from build123d import *

# Parameters (mm, degrees)
F0_W     = 5
F0_H     = 30
F1_DEPTH = 6
F2_R     = 0.948442
F3_DEPTH = 1
F4_R     = 1.863501
F5_DEPTH = 5.001


with BuildPart() as f1:
    # F0 (on Front) → F1 (new body)
    with BuildSketch(Plane.XZ):
        with Locations((2.5, 0)):
            Rectangle(F0_W, F0_H)
    extrude(amount=F1_DEPTH)

    # F2 (on face) → F3 (cut)
    with BuildSketch(Plane.YZ.offset(5)):
        with Locations((-2.562478, 8.886208)):
            Circle(F2_R)
    extrude(amount=-F3_DEPTH, mode=Mode.SUBTRACT)

    # F4 (on face) → F5 (cut, through all)
    with BuildSketch(Plane.YZ.offset(5)):
        with Locations((-2.708179, 2.568147)):
            Circle(F4_R)
    extrude(amount=-F5_DEPTH, mode=Mode.SUBTRACT)


solid = f1.part
Read the model definition and answer for the solid it produces. Units are mm, in the model's axes. Round coordinates to 2 decimals unless told otherwise and drop trailing zeros. Order: outer loops, then holes, each group sorted by start corner. A loop starts at its lowest first (then second) coordinate and runs counter-clockwise, first axis right, second up.
1) The part is cut by section B-B on x = 4.6. Write down the section's boundary in (y, z), plus the area to 3 significant figures.
2) Straight lines are drawn through the part: L1, parallel to X at y = -2.75, z = 8.5; L2, parallel to Y at x = 2.55, z = 2.5; L3, parallel to Z at x = 1.4, y = -3.55. For each, find the intervals that lie inside material, in ascending order.
3) The part is cut by section C-C on x = 3.5. Write down the section's boundary in (y, z).
4) Flat-ended cylindrical pins translate along their axes: pin 1 (0.6 mm diameter, centred on y = -2.5, z = 9, fed in from +X); pin 2 (3 mm diameter, centred on y = -2.71, z = 2.57, fed in from +X). Find the tip coordinate at first contact, or state that the pin passes through.
5) The mould has two halves that part along Y. Classify faces 1 (the face through (2, 0, 0)), 2 (the face through (0, -3, 0)), 3 (the face through (4.51, -2.77, 7.96)), 4 (the face through (4, -3, 9)): released by +Y, released by -Y, zero draft, split by the parting line, or undercut.
6) The part is cut by section A-A on y = -2.85. Write down the section's boundary in (x, z), plus the area to 3 significant figures.
Resolved:
1. outline: (-6, -15) - (0, -15) - (0, 15) - (-6, 15) - close; hole circle Ø3.73 at (-2.71, 2.57); hole circle Ø1.9 at (-2.56, 8.89)
1. area: 166 mm2
2. L1: x = 0 to 4
2. L2: y = -6 to -4.57, -0.85 to 0
2. L3: z = -15 to 0.91, 4.23 to 15
3. outline: (-6, -15) - (0, -15) - (0, 15) - (-6, 15) - close; hole circle Ø3.73 at (-2.71, 2.57)
4. pin 1: stops at x = 4
4. pin 2: passes through
5. face 1: released by +Y
5. face 2: zero draft
5. face 3: undercut
5. face 4: undercut
6. outline: (0, -15) - (5, -15) - (5, 0.71) - (0, 0.71) - close; (0, 4.43) - (5, 4.43) - (5, 7.98) - (4, 7.98) - (4, 9.79) - (5, 9.79) - (5, 15) - (0, 15) - close
6. area: 130 mm2
